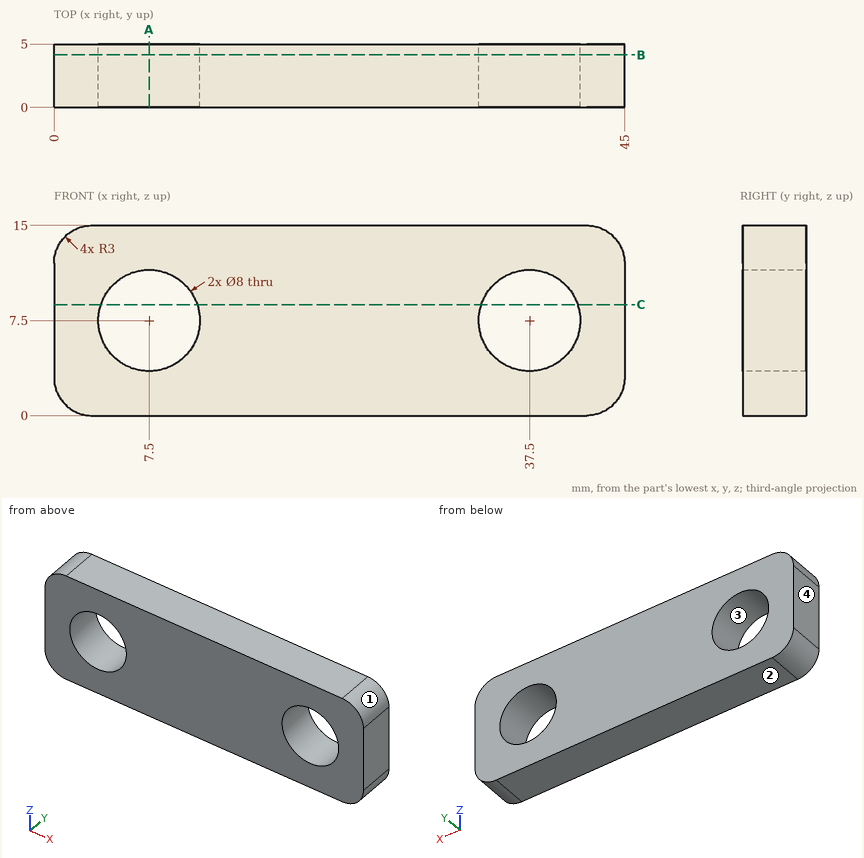
For this review, use the dimensioned drawing (mm, ordinates from the lowest corner) and the shaded views. Give positions to 0.01 mm unless a question says otherwise; leave off trailing zeros. Order: outer loops, then holes, each group sorted by start corner. A loop starts at its lowest first (then second) coordinate and runs counter-clockwise, first axis right, second up. Notation, with made-up numbers: (70, -5.5) - (108, -5.5) arc R26 cw to (108, 30.5) - close; hole circle Ø1 at (0.5, -2.5). An arc over 180 degrees is marked (long way). Use CSV: the item, a comma, the result in double quotes. Start each with the question number.
Q1. We need section A-A, the plane x = 7.5. Write out the cut boundary in (y, z).
Q2. We need section B-B, the plane y = 4.15. Write out the cut boundary in (x, z), and give its area (3 significant figures).
Q3. To check wall thickness, follow line 1 along X through (y, z) = (1.95, 7.5); line 2 along Z through (x, y) = (37.5, 1.8); line 3 along X through (y, z) = (1.6, 10.5). State the ranges of each line that lie inside material, in increasing order. Write a range as [from, to].
Q4. We need section C-C, the plane z = 8.75. Write out the cut boundary in (x, y).
Q5. The part is to be moulded in two halves that separate along Z. For the marked faces 1, 2, 3 and 4, say which applies: +Z half, -Z half, draft (parallel to the pull), parting line (faces both ways), or undercut.
Outcome:
1,outline,"(0, 0) - (5, 0) - (5, 3.5) - (0, 3.5) - close; (0, 11.5) - (5, 11.5) - (5, 15) - (0, 15) - close"
2,outline,"(0, 3) arc R3 ccw to (3, 0) - (42, 0) arc R3 ccw to (45, 3) - (45, 12) arc R3 ccw to (42, 15) - (3, 15) arc R3 ccw to (0, 12) - close; hole circle Ø8 at (7.5, 7.5); hole circle Ø8 at (37.5, 7.5)"
2,area,"567 mm^2"
3,line 1,"x = [0, 3.5], [11.5, 33.5], [41.5, 45]"
3,line 2,"z = [0, 3.5], [11.5, 15]"
3,line 3,"x = [0, 4.85], [10.15, 34.85], [40.15, 45]"
4,outline,"(0, 0) - (3.7, 0) - (3.7, 5) - (0, 5) - close; (11.3, 0) - (33.7, 0) - (33.7, 5) - (11.3, 5) - close; (41.3, 0) - (45, 0) - (45, 5) - (41.3, 5) - close"
5,face 1,"+Z half"
5,face 2,"-Z half"
5,face 3,"undercut"
5,face 4,"draft"
